Design review of the part built by this model. Coordinates are the model's own, in mm. A direction names the side the tool comes from. Give positions to 0.01 mm unless a question says otherwise; leave off trailing zeros. Order: outer loops, then holes, each group sorted by start corner. A loop starts at its lowest first (then second) coordinate and runs counter-clockwise, first axis right, second up. Notation, with made-up numbers: (6.5, -24) - (30.5, -24) arc R28 ccw to (30.5, 11) - close; hole circle Ø9 at (52.25, -4.75). An arc over 180 degrees is marked (long way). Write each question's results on one line, items separated by ' | '. Start each with the question number.
```python
from build123d import *

# Parameters (mm, degrees)
SKETCH1_W           = 25.4
SKETCH1_H           = 25.4
BOSS_EXTRUDE1_DEPTH = 1.016
SKETCH2_W           = 22.0218
SKETCH2_H           = 5.4102
BOSS_EXTRUDE2_DEPTH = 2.667
SKETCH3_W           = 8.0264
SKETCH3_H           = 7.9756
BOSS_EXTRUDE3_DEPTH = 3.58902


with BuildPart() as part:
    # Sketch1 → Boss-Extrude1 (new body)
    with BuildSketch(Plane.XY):
        Rectangle(SKETCH1_W, SKETCH1_H)
    extrude(amount=BOSS_EXTRUDE1_DEPTH)

    # Sketch2 → Boss-Extrude2 (add)
    with BuildSketch(Plane.XY.offset(1.016)):
        with Locations((0, -9.9949)):
            Rectangle(SKETCH2_W, SKETCH2_H)
    extrude(amount=BOSS_EXTRUDE2_DEPTH)

    # Sketch3 → Boss-Extrude3 (add)
    with BuildSketch(Plane(origin=(0, 0, 0), x_dir=(-1, 0, 0), z_dir=(0, 0, -1))):
        with Locations((0, -3.4798)):
            Rectangle(SKETCH3_W, SKETCH3_H)
    extrude(amount=BOSS_EXTRUDE3_DEPTH)


solid = part.part
```
Q1. Add section D-D (x = 9.75). Give the boundary of the cut face in (y, z).
Q2. Add section A-A (x = 0.75). Give the boundary of the cut face in (y, z), plus the area to 3 significant figures.
Q3. Add section B-B (y = 0). Give the boundary of the cut face in (x, z), plus the area to 3 significant figures.
Q4. Insertion check: pin 1 Ø1 at (x, z) = (-7.5, -1.5) entering from -Y; pin 2 Ø3 at (x, z) = (1.5, -2) entering from +Y; pin 3 Ø1.8 at (y, z) = (-3, -1) entering from -X; pin 4 Ø1.3 at (y, z) = (-10, 2.5) entering from -X. Each pin has a flat end and moves straight along its axis. Give the tip position at first contact, or say it passes through.
Q5. Machinability: for faces 1 (the flat face through (11.011, -10, 2)), 2 (the flat face through (-11.011, -10, 2)), 3 (the flat face through (4.013, -4, -2)), which of the approach directions +Z, -Z, +X, -X, +Y, -Y give a long, thin tool a straight path to every point of the face, cutting with its end or side? Answer none if there is none.
Q6. Add section C-C (z = 3.25). Give the boundary of the cut face in (x, y).
Q7. For line 1 (Y direction, x = 2.5, z = -0.5); line 2 (X direction, y = -5.25, z = -2.25); line 3 (Z direction, x = -11.5, y = -6.75), list the stretches that pass through material, from the lowest coordinate up. Write a range as [from, to].
Verdict:
1) outline: (-12.7, 0) - (12.7, 0) - (12.7, 1.02) - (-7.29, 1.02) - (-7.29, 3.68) - (-12.7, 3.68) - close
2) outline: (-12.7, 0) - (-7.47, 0) - (-7.47, -3.59) - (0.51, -3.59) - (0.51, 0) - (12.7, 0) - (12.7, 1.02) - (-7.29, 1.02) - (-7.29, 3.68) - (-12.7, 3.68) - close | area: 68.9 mm2
3) outline: (-12.7, 0) - (-4.01, 0) - (-4.01, -3.59) - (4.01, -3.59) - (4.01, 0) - (12.7, 0) - (12.7, 1.02) - (-12.7, 1.02) - close | area: 54.6 mm2
4) pin 1: passes through | pin 2: stops at y = 0.51 | pin 3: stops at x = -4.01 | pin 4: stops at x = -11.01
5) face 1: +Z, +X, +Y, -Y | face 2: +Z, -X, +Y, -Y | face 3: -Z, +X, +Y, -Y
6) outline: (-11.01, -12.7) - (11.01, -12.7) - (11.01, -7.29) - (-11.01, -7.29) - close
7) line 1: y = [-7.47, 0.51] | line 2: x = [-4.01, 4.01] | line 3: z = [0, 1.02]
